Design review of the part built by this model. Coordinates are the model's own, in mm. Face numbers are marked on the shaded views. A direction names the side the tool comes from. Give positions to 0.01 mm unless a question says otherwise; leave off trailing zeros. Order: outer loops, then holes, each group sorted by start corner. A loop starts at its lowest first (then second) coordinate and runs counter-clockwise, first axis right, second up. Notation, with made-up numbers: M -25,26 L 7,26 A24 cw 7,58 Z; hole C 11.25,4 d3. An arc over 180 degrees is marked long. Answer as a JSON object with one key per item and string values.
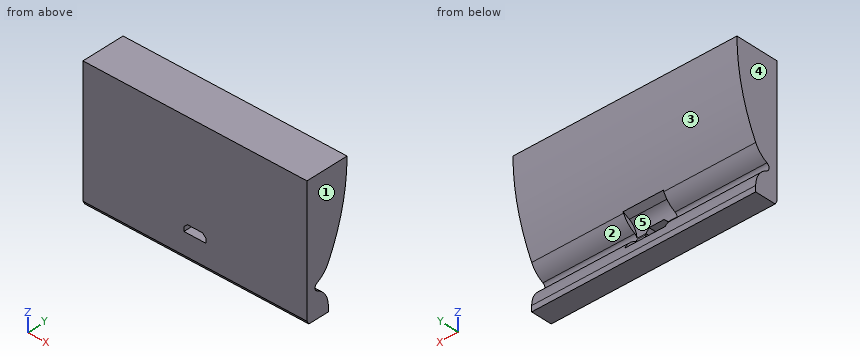
from build123d import *

# Parameters (mm, degrees)
EXTRUDE_1509_DEPTH      = 38.971143
EXTRUDE_1509_DEPTH_BACK = 38.971143
USB_REACH               = 62.065
CUT_EXTRUDE_2243_DEPTH  = 7


with BuildPart() as part:
    # Эскиз1 → Extrude 1509 (new, two sides: drawn at the far end of the back side and taken through both)
    with BuildSketch(Plane(origin=(0, 0, 0), x_dir=(0, 0, -1), z_dir=(1, 0, 0)).offset(-EXTRUDE_1509_DEPTH_BACK)):
        with BuildLine():
            Line((0, 60.5), (-2, 60.5))
            ThreePointArc((-2, 60.5), (-5.97996079, 59.358562264), (-8.75, 56.28125))
            ThreePointArc((-8.75, 56.28125), (-10, 55.5), (-11.25, 56.28125))
            ThreePointArc((-11.25, 56.28125), (-12.988798615, 58.733904838), (-15.421871621, 60.5))
            ThreePointArc((-15.421871621, 60.5), (-29.802420601, 65.726159332), (-45, 67.5))
            Line((-45, 67.5), (-45, 52.5))
            Line((-45, 52.5), (-1.212435565, 52.5))
            Line((-1.212435565, 52.5), (0, 53.2))
            Line((0, 53.2), (0, 60.5))
        make_face()
    extrude(amount=EXTRUDE_1509_DEPTH + EXTRUDE_1509_DEPTH_BACK)

    # Эскиз3 → Вырез под USB (cut, up to next)
    with BuildSketch(Plane(origin=(0, 60.5, 0), x_dir=(1, 0, 0), z_dir=(0, 1, 0)), mode=Mode.PRIVATE) as usb_sk1:
        Polygon((3.85, -8.65), (-3.85, -8.65), (-3.85, -10.15), (-2.65, -11.35), (2.65, -11.35), (3.85, -10.15), align=None)
    usb_tool1 = extrude(usb_sk1.sketch, amount=-USB_REACH, mode=Mode.PRIVATE) & part.part
    add(usb_tool1.solids().sort_by_distance((0, 60.5, 9.929302))[0], mode=Mode.SUBTRACT)

    # Эскиз4 → Cut-Extrude 2243 (cut, symmetric)
    with BuildSketch(Plane(origin=(0, 0, 0), x_dir=(0, 0, -1), z_dir=(1, 0, 0))):
        with BuildLine():
            Line((-5.65, 58.328664085), (-1.315214811, 67.278875413))
            Line((-1.315214811, 67.278875413), (-18.984785189, 67.278875413))
            Line((-18.984785189, 67.278875413), (-14.65, 58.328664085))
            ThreePointArc((-14.65, 58.328664085), (-10.15, 55.508113557), (-5.65, 58.328664085))
        make_face()
    extrude(amount=CUT_EXTRUDE_2243_DEPTH, both=True, mode=Mode.SUBTRACT)


solid = part.part
(1) We need section B-B (z = 7). Write out the cut boundary in (x, y).
Checked values:
{"outline": "M -38.97,52.5 L 38.97,52.5 L 38.97,58.59 L 7,58.59 L 7,56.63 L -7,56.63 L -7,58.59 L -38.97,58.59 Z"}
(2) We need section D-D (z = 39). Write out the cut boundary in (x, y), plus the area to 3 significant figures.
Checked values:
{"outline": "M -38.97,52.5 L 38.97,52.5 L 38.97,67.23 L -38.97,67.23 Z", "area": "1,150 mm^2"}
(3) We need section A-A (x = 30). Write out the cut boundary in (y, z).
Checked values:
{"outline": "M 52.5,1.21 L 53.2,0 L 60.5,0 L 60.5,2 A7.51 ccw 56.28,8.75 A1.39 cw 56.28,11.25 A9.26 ccw 60.5,15.42 A65.99 ccw 67.5,45 L 52.5,45 Z"}
(4) Draft analysis for pull direction Z (two halves, no side actions). For the marked faces 3, 4 and 5, state which applies: +Z half, -Z half, draft (parallel to the pull), parting line (faces both ways), or undercut.
Checked values:
{"face 3": "-Z half", "face 4": "draft", "face 5": "undercut"}
(5) Insertion check: pin 1 (1.6 mm diameter, centred on x = -12, z = 1, fed in from +Y); pin 2 (2 mm diameter, centred on x = -3, y = 55.5, fed in from -Z). Each pin has a flat end and moves straight along its axis. Give the tip position at first contact, or say it passes through.
Checked values:
{"pin 1": "stops at y = 60.5", "pin 2": "stops at z = 0"}
(6) We need section C-C (y = 63). Write out the cut boundary in (x, z), plus the area to 3 significant figures.
Checked values:
{"outline": "M -38.97,21.05 L 38.97,21.05 L 38.97,45 L -38.97,45 Z", "area": "1,870 mm^2"}
(7) Tool access review of the marked faces 1 and 2: name each direction out of +Z, -Z, +X, -X, +Y, -Y from which nothing blocks a thin tool from reaching the whole face with its end or side.
Checked values:
{"face 1": "+Z, -Z, +X, +Y, -Y", "face 2": "+X, -X, +Y"}
(8) To check wall thickness, follow L1, parallel to Z at x = -35, y = 56.25; L2, parallel to Z at x = -2, y = 57.75; L3, parallel to Y at x = -23, z = 17.5. State the ranges of each line that lie inside material, in increasing order. Write a range as from..to.
Checked values:
{"L1": "z = 0..8.77, 11.23..45", "L2": "z = 0..5.98, 14.32..45", "L3": "y = 52.5..61.5"}
